from build123d import *

# Parameters (mm, degrees)
EXTRUDE_4_DEPTH = 15
SKETCH_10_R     = 15
EXTRUDE_5_DEPTH = 17


with BuildPart() as part:
    # ｽｹｯﾁ2 → ﾎﾞｽ - 押し出し4 (new body)
    with BuildSketch(Plane(origin=(0, 0, 0), x_dir=(1, 0, 0), z_dir=(0, 1, 0))):
        with BuildLine():
            ThreePointArc((-53.82643789, -36.437818048), (-56.846261527, -34.367935813), (-60.466933112, -34.910600109))
            Line((-60.466933112, -34.910600109), (-64.807406984, -37.416573868))
            ThreePointArc((-64.807406984, -37.416573868), (-67.177509772, -40.614402853), (-66.461234116, -44.529814279))
            ThreePointArc((-66.461234116, -44.529814279), (49.665387485, -62.716419588), (58.57572973, 54.487465409))
            Line((58.57572973, 54.487465409), (57.289371136, 55.838409315))
            Line((57.289371136, 55.838409315), (25.911523347, 88.791671712))
            ThreePointArc((25.911523347, 88.791671712), (19.306695871, 93.382511176), (11.427401304, 95))
            Line((11.427401304, 95), (0, 95))
            ThreePointArc((0, 95), (-15, 80), (0, 65))
            ThreePointArc((0, 65), (57.41714976, -30.467538684), (-53.82643789, -36.437818048))
        make_face()
    extrude(amount=EXTRUDE_4_DEPTH)

    # ｽｹｯﾁ10 → ﾎﾞｽ - 押し出し5 (add)
    with BuildSketch(Plane(origin=(0, 15, 0), x_dir=(1, 0, 0), z_dir=(0, 1, 0))):
        with Locations(Location((0, 79.906692584, 0), (0, 0, 179.821795675))):
            Circle(SKETCH_10_R)
    extrude(amount=EXTRUDE_5_DEPTH)


solid = part.part
Geometry: final body of the model. Coordinates: model frame, mm. A direction names the side the tool comes from. Round coordinates to 2 decimals unless told otherwise and drop trailing zeros. Write each loop counter-clockwise with the first axis right and the second up, starting at its lowest first coordinate (ties: lowest second). Pieces come first, ordered by that corner, then holes. Notation, with made-up numbers: M -6,-39.5 L 47,-39.5 A18 ccw 47,-9.5 Z; hole C 71,34.25 d10. An arc over 180 degrees is marked long. Write item = value, one per line.
Item 1: Material intervals for line 1 along Z through (x, y) = (0, 7.5); line 2 along Z through (x, y) = (-3, 12); line 3 along Y through (x, z) = (58.5, -40.5), sorted ascending. Write a range as [from, to].
Findings:
line_1 = [-95, -65], [65, 80]
line_2 = [-94.7, -65.3], [64.93, 79.94]
line_3 = [0, 15]
Item 2: Pull-direction query (Z, two-part tool) for faces 1 (the face through (-67.164, 7.395, 40.559)), 2 (the face through (-15, 7, -80)), 3 (the face through (-62.61, 7.4, 36.15)); classes: pulls with the +Z half, pulls with the -Z half, needs draft (parallel to the pull), parting line crosses it, or undercut.
Findings:
face_1 = parting line crosses it
face_2 = undercut
face_3 = pulls with the -Z half
Item 3: Pin query (flat end, axial travel): P1, Ø5, axis at x = 32.5, y = 10.5, coming from the +Z side; P2, Ø6, axis at y = 7, z = 50, coming from the -X side; P3, Ø8, axis at x = 64.5, z = 54.5, coming from the -Y side; P4, Ø12, axis at x = 35.5, y = 10.5, coming from the -Z side. Return the tip coordinate at first contact, or that it passes through.
Findings:
P1 = 74.16
P2 = -64.74
P3 = through
P4 = -85.02
Item 4: Section query B-B on x = -5. Return loops of the section in (y, z), then the cut area to 3 significant figures.
Findings:
outline = M 0,-94.14 L 15,-94.14 L 15,-94.05 L 32,-94.05 L 32,-65.76 L 15,-65.76 L 15,-65.86 L 0,-65.86 Z; M 0,64.81 L 15,64.81 L 15,79.84 L 0,79.84 Z
area = 1,130 mm^2
Item 5: Section query A-A on z = 61.5. Return loops of the section in (x, y).
Findings:
outline = M -51.16,0 L -21.04,0 L -21.04,15 L -51.16,15 Z; M 21.04,0 L 51.16,0 L 51.16,15 L 21.04,15 Z
Item 6: Access query for faces 4 (the face through (3.3, 23.38, -94.54)), 5 (the face through (0, 32, -80)). Directions: +Z, -Z, +X, -X, +Y, -Y. A direction counts if a zero-diameter tool reaches every point of the face in a straight line with its end or side. Return the directions, or none.
Findings:
face_4 = +Y
face_5 = +Z, -Z, +X, -X, +Y
Item 7: Section query C-C on y = 7. Return loops of the section in (x, z), then the cut area to 3 significant figures.
Findings:
outline = M -66.46,44.53 A5 ccw -64.81,37.42 L -60.47,34.91 A5 ccw -53.83,36.44 A65 cw long 0,-65 A15 ccw 0,-95 L 11.43,-95 A20 ccw 25.91,-88.79 L 58.58,-54.49 A80 ccw long Z
area = 5,450 mm^2
